Here's how the part is built. I have some questions about the finished solid (model axes, mm). A direction names the side the tool comes from. Round coordinates to 2 decimals unless told otherwise and drop trailing zeros. Loops run counter-clockwise (first coordinate to the right, second up) from the corner with the lowest first, then second, coordinate; pieces in that order, holes last. Notation, with made-up numbers: (36, 5) - (78, 5) arc R21 cw to (78, 29) - close; hole circle Ø9 at (-4, -35). An arc over 180 degrees is marked (long way). Answer as a JSON object with one key per item and string values. Group by question number.
1) I want a section at B-B, the plane z = 0. Please give me the cut outline in (x, y).
2) If I drill on line 1 along X through (y, z) = (4.75, -16); line 2 along Y through (x, z) = (-18, -3); line 3 along Z through (x, y) = (28, 19.3), over which ranges is the centre line in solid material (lowest first)? Write a range as [from, to].
3) I want a section at A-A, the plane x = -20. Please give me the cut outline in (y, z), then the cut area to 3 significant figures.
4) Which directions (+Z, -Z, +X, -X, +Y, -Y) give clear straight access to the entire face, cutting with the end or side of a thin tool? Please do faces 1 (the face through (-11.82, 19.97, -4.1)), 2 (the face through (12, 5, -19.25)), 3 (the face through (11.82, 19.97, -4.1)), 4 (the face through (11.25, 17, 0)).
5) If we mould it in two halves opening along Z, with no side actions, what happens to faces 5 (the face through (0, 10, -1)), 6 (the face through (-22, 20, 3.5)), 7 (the face through (0, 18, -11.25))? For each: pulls with the +Z half, pulls with the -Z half, needs draft (parallel to the pull), parting line crosses it, or undercut.
6) I want a section at C-C, the plane y = 20. Please give me the cut outline in (x, z).
7) I want a section at D-D, the plane y = 4. Please give me the cut outline in (x, z).
8) Will these pins go through, and if not, where does the flat tip stop? P1, Ø2, axis at x = 4, z = 16, coming from the +Y side; P2, Ø19, axis at x = -1.5, z = 4, coming from the -Y side; P3, Ø3.5, axis at y = 6.5, z = 4.5, coming from the -X side; P4, Ø3.5, axis at x = 28, z = 0, coming from the -Y side.
from build123d import *

# Parameters (mm, degrees)
SKETCH1_W           = 42.5
SKETCH1_H           = 42.5
SKETCH1_W_2         = 38.5
SKETCH1_H_2         = 38.5
BOSS_EXTRUDE1_DEPTH = 10
SKETCH2_W           = 42.5
SKETCH2_H           = 42.5
BOSS_EXTRUDE2_DEPTH = 2
SKETCH3_W           = 4
SKETCH3_H           = 2
CUT_EXTRUDE1_DEPTH  = 10
SKETCH5_W           = 22.5
SKETCH5_H           = 22.5
BOSS_EXTRUDE3_DEPTH = 10
BOSS_EXTRUDE4_DEPTH = 4
FILLET1_R           = 2
FILLET2_R           = 3


with BuildPart() as part:
    # Sketch1 → Boss-Extrude1 (new body)
    with BuildSketch(Plane(origin=(0, 0, 0), x_dir=(1, 0, 0), z_dir=(0, 1, 0))):
        Rectangle(SKETCH1_W, SKETCH1_H)
        Rectangle(SKETCH1_W_2, SKETCH1_H_2, mode=Mode.SUBTRACT)
    extrude(amount=BOSS_EXTRUDE1_DEPTH)

    # Sketch2 → Boss-Extrude2 (add)
    with BuildSketch(Plane(origin=(0, 10, 0), x_dir=(1, 0, 0), z_dir=(0, 1, 0))):
        Rectangle(SKETCH2_W, SKETCH2_H)
    extrude(amount=BOSS_EXTRUDE2_DEPTH)

    # Sketch3 → Cut-Extrude1 (cut)
    with BuildSketch(Plane.XZ):
        with Locations((-2, -20.25)):
            Rectangle(SKETCH3_W, SKETCH3_H)
        with Locations((2, -20.25)):
            Rectangle(SKETCH3_W, SKETCH3_H)
    extrude(amount=-CUT_EXTRUDE1_DEPTH, mode=Mode.SUBTRACT)

    # Sketch5 → Boss-Extrude3 (add)
    with BuildSketch(Plane(origin=(0, 12, 0), x_dir=(1, 0, 0), z_dir=(0, 1, 0))):
        Rectangle(SKETCH5_W, SKETCH5_H)
    extrude(amount=BOSS_EXTRUDE3_DEPTH)

    # Sketch6 → Boss-Extrude4 (add)
    with BuildSketch(Plane(origin=(0, 22, 0), x_dir=(1, 0, 0), z_dir=(0, 1, 0))):
        with BuildLine():
            Line((32, 0), (29.85, 0))
            ThreePointArc((29.85, 0), (28, -1.85), (26.15, 0))
            Line((26.15, 0), (11.25, 0))
            Line((11.25, 0), (11.25, -3.5))
            Line((11.25, -3.5), (32, -3.5))
            Line((32, -3.5), (32, 0))
        make_face()
        with BuildLine():
            ThreePointArc((26.15, 0), (28, 1.85), (29.85, 0))
            Line((29.85, 0), (32, 0))
            Line((32, 0), (32, 3.5))
            Line((32, 3.5), (11.25, 3.5))
            Line((11.25, 3.5), (11.25, 0))
            Line((11.25, 0), (26.15, 0))
        make_face()
    boss_extrude4 = extrude(amount=-BOSS_EXTRUDE4_DEPTH)

    # Mirror2: Boss-Extrude4 across plane
    add(boss_extrude4.mirror(Plane(origin=(0, 0, 0), x_dir=(0, 0, 1), z_dir=(1, 0, 0))))

    # Fillet1
    fillet1_edges = [part.edges().sort_by_distance(p)[0] for p in [
        (0, 12, -11.25),
        (-11.25, 12, 0),
        (0, 12, 11.25),
        (11.25, 12, 0),
        (11.25, 20, -3.5),
        (32, 20, -3.5),
        (32, 20, 3.5),
        (11.25, 20, 3.5),
        (-32, 20, -3.5),
        (-11.25, 20, -3.5),
        (-11.25, 20, 3.5),
        (-32, 20, 3.5),
    ]]
    fillet(fillet1_edges, radius=FILLET1_R)

    # Fillet2
    fillet2_edges = [part.edges().sort_by_distance(p)[0] for p in [
        (4, 0, -20.25),
        (-4, 0, -20.25),
    ]]
    fillet(fillet2_edges, radius=FILLET2_R)


solid = part.part
Outcome:
{
 "1": {"outline": "(-32, 18) - (-29.85, 18) - (-29.85, 22) - (-32, 22) - close; (-26.15, 18) - (-11.25, 18) - (-11.25, 14) arc R2 cw to (-13.25, 12) - (-21.25, 12) - (-21.25, 0) - (-19.25, 0) - (-19.25, 10) - (19.25, 10) - (19.25, 0) - (21.25, 0) - (21.25, 12) - (13.25, 12) arc R2 cw to (11.25, 14) - (11.25, 18) - (26.15, 18) - (26.15, 22) - (-26.15, 22) - close; (29.85, 18) - (32, 18) - (32, 22) - (29.85, 22) - close"},
 "2": {"line 1": "[-21.25, -19.25], [19.25, 21.25]", "line 2": "[10, 12], [18, 22]", "line 3": "[-3.5, -1.85], [1.85, 3.5]"},
 "3": {"outline": "(0, -21.25) - (12, -21.25) - (12, 21.25) - (0, 21.25) - close; (18, -3.5) - (22, -3.5) - (22, 3.5) - (18, 3.5) - close", "area": "538 mm^2"},
 "4": {"face 1": "-Z, -X, +Y", "face 2": "-Y", "face 3": "-Z, +X, +Y", "face 4": "+X"},
 "5": {"face 5": "undercut", "face 6": "pulls with the +Z half", "face 7": "pulls with the -Z half"},
 "6": {"outline": "(-32, -1.5) arc R2 ccw to (-30, -3.5) - (-13.25, -3.5) arc R2 cw to (-11.25, -5.5) - (-11.25, -11.25) - (11.25, -11.25) - (11.25, -5.5) arc R2 cw to (13.25, -3.5) - (30, -3.5) arc R2 ccw to (32, -1.5) - (32, 1.5) arc R2 ccw to (30, 3.5) - (13.25, 3.5) arc R2 cw to (11.25, 5.5) - (11.25, 11.25) - (-11.25, 11.25) - (-11.25, 5.5) arc R2 cw to (-13.25, 3.5) - (-30, 3.5) arc R2 ccw to (-32, 1.5) - close; hole circle Ø3.7 at (-28, 0); hole circle Ø3.7 at (28, 0)"},
 "7": {"outline": "(-21.25, -21.25) - (-4, -21.25) - (-4, -19.25) - (-19.25, -19.25) - (-19.25, 19.25) - (19.25, 19.25) - (19.25, -19.25) - (4, -19.25) - (4, -21.25) - (21.25, -21.25) - (21.25, 21.25) - (-21.25, 21.25) - close"},
 "8": {"P1": "y = 12", "P2": "y = 10", "P3": "x = -21.25", "P4": "through"}
}
